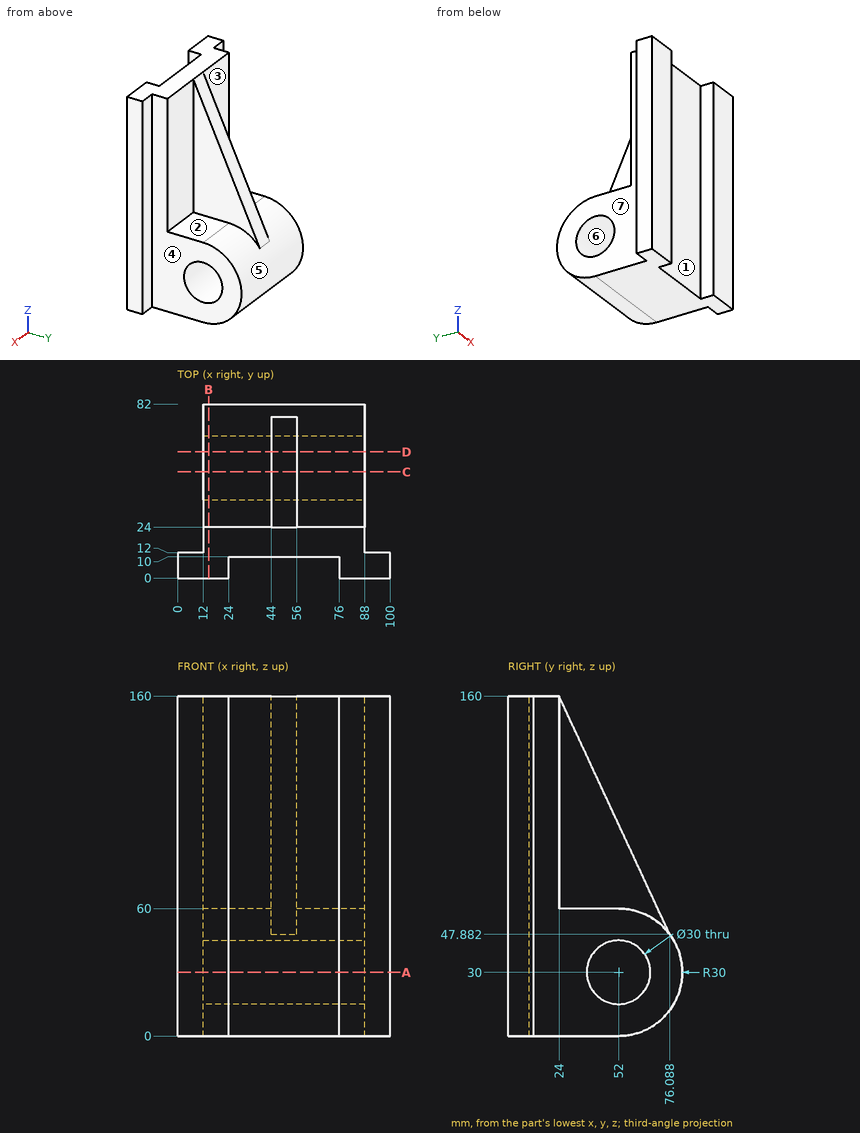
Geometry check sheet. Reference: drawing and pictorial views, mm from the part's lowest x, y, z. A direction names the side the tool comes from. Give positions to 0.01 mm unless a question says otherwise; leave off trailing zeros. Loops run counter-clockwise (first coordinate to the right, second up) from the corner with the lowest first, then second, coordinate; pieces in that order, holes last.
1. Mould release check, pull along Y, two halves, no side actions. Record for the marked faces 5, 6 and 7: released by +Y, released by -Y, zero draft, split by the parting line, or undercut.
2. Set-up check for the marked faces 1, 2, 3 and 4: record each of +Z, -Z, +X, -X, +Y, -Y from which the full face is reachable in a straight line by a thin tool's end or side.
3. Go/stop test with flat-tipped pins: pin 1 Ø5 at (x, z) = (45.5, 104) entering from -Y; pin 2 Ø1 at (x, z) = (76.5, 144) entering from +Y; pin 3 Ø15.5 at (y, z) = (50, 93) entering from -X. Record where each tip stops, or that it passes through.
4. Thickness scan on line 1 (Y direction, x = 69.5, z = 30); line 2 (Z direction, x = 68, y = 52.5); line 3 (Y direction, x = 27, z = 118). Record the ranges inside material, lowest first.
5. Section check B-B, the plane x = 14.5. Enter the section's corners in (y, z).
6. Section check A-A, the plane z = 30. Enter the section's corners in (x, y), then the cut area to 3 significant figures.
7. Section check D-D, the plane y = 59.5. Enter the section's corners in (x, z), then the cut area to 4 significant figures.
8. Section check C-C, the plane y = 50. Enter the section's corners in (x, z).
Geometry says:
1. face 5: released by +Y
1. face 6: undercut
1. face 7: zero draft
2. face 1: +Z, -Z, -Y
2. face 2: +Z, +X, +Y
2. face 3: +Z, -X, +Y
2. face 4: +Z, -Z, +X, +Y
3. pin 1: stops at y = 10
3. pin 2: stops at y = 24
3. pin 3: stops at x = 44
4. line 1: y = 10 to 37, 67 to 82
4. line 2: z = 0 to 15.01, 44.99 to 60
4. line 3: y = 10 to 24
5. outline: (0, 0) - (52, 0) arc R30 ccw to (52, 60) - (24, 60) - (24, 160) - (0, 160) - close; hole circle Ø30 at (52, 30)
6. outline: (0, 0) - (24, 0) - (24, 10) - (76, 10) - (76, 0) - (100, 0) - (100, 12) - (88, 12) - (88, 37) - (12, 37) - (12, 12) - (0, 12) - close; (12, 67) - (88, 67) - (88, 82) - (12, 82) - close
6. area: 3,720 mm2
7. outline: (12, 0.95) - (88, 0.95) - (88, 17.01) - (12, 17.01) - close; (12, 42.99) - (88, 42.99) - (88, 59.05) - (56, 59.05) - (56, 83.59) - (44, 83.59) - (44, 59.05) - (12, 59.05) - close
7. area: 2,735 mm2
8. outline: (12, 0) - (88, 0) - (88, 15.13) - (12, 15.13) - close; (12, 44.87) - (88, 44.87) - (88, 60) - (56, 60) - (56, 104.04) - (44, 104.04) - (44, 60) - (12, 60) - close
